The listing builds one solid part. Answer for the finished solid, in the listing's coordinates (mm). A direction names the side the tool comes from. Give positions to 0.01 mm unless a question says otherwise; leave off trailing zeros. Order: outer loops, then holes, each group sorted by start corner. A loop starts at its lowest first (then second) coordinate and runs counter-clockwise, first axis right, second up. Notation, with made-up numbers: (-31.75, -40) - (3.25, -40) arc R34 ccw to (3.25, -4) - close; hole circle Ø11 at (50.5, -8.5). An arc over 180 degrees is marked (long way). Answer as a JSON object with one key per item and string values. Group by question number.
Q1. For faces 1 (the face through (11.923, -3.755, -80.14)), 2 (the face through (11.923, 3.755, 9.86)), 3 (the face through (-0.342, 52.497, -65.07)), determine the directions among +Z, -Z, +X, -X, +Y, -Y from which every point of the face is accessible in a straight line to the end or side of a thin tool.
Q2. A cutting plane is placed at D-D, the plane y = 35. Give the vertices of the cut face in (x, z), and give its area (3 significant figures).
Q3. The mould has two halves that part along Z. Classify faces 4 (the face through (-10, -9, 0)), 5 (the face through (-1.627, 22.606, -34.65)), 6 (the face through (20.188, 21.289, -4.93)), 7 (the face through (1, -9, -10)): released by +Z, released by -Z, zero draft, split by the parting line, or undercut.
Q4. A cutting plane is placed at A-A, the plane y = -2. Give the vertices of the cut face in (x, z).
Q5. A cutting plane is placed at B-B, the plane x = 19.5. Give the vertices of the cut face in (y, z).
Q6. Consider line 1 (Z direction, x = 1, y = 5); line 2 (Z direction, x = 16, y = -31); line 3 (Z direction, x = -2, y = 24). Determine where each line is inside the solid, lowest interval first.
Q7. A cutting plane is placed at C-C, the plane x = 0. Give the vertices of the cut face in (y, z).
Q8. Given pin 1 (8 mm diameter, centred on x = 42, z = -7.5, fed in from +Y); pin 2 (2 mm diameter, centred on x = -12, y = -38, fed in from +Z); pin 3 (12 mm diameter, centred on y = -24.5, z = -74.5, fed in from -X), each flat-ended and moving along its own axis, determine where each tip first touches the part or whether it passes through.
from build123d import *

# Parameters (mm, degrees)
SKETCH2_R           = 12.5
BOSS_EXTRUDE1_DEPTH = 20
BOSS_EXTRUDE2_DEPTH = 10
FILLET1_R           = 5
SKETCH4_R           = 12.5
BOSS_EXTRUDE3_DEPTH = 50
BOSS_EXTRUDE4_START = 20
SKETCH5_R           = 12.5
BOSS_EXTRUDE4_DEPTH = 20


with BuildPart() as part:
    # Sketch2 → Boss-Extrude1 (new body)
    with BuildSketch(Plane.XY):
        Circle(SKETCH2_R)
    extrude(amount=BOSS_EXTRUDE1_DEPTH)

    # Sketch3 → Boss-Extrude2 (add)
    with BuildSketch(Plane.XY):
        with BuildLine():
            Line((-49.999953659, -0.068074118), (-23.953413336, -0.068074118))
            Line((-23.953413336, -0.068074118), (-17.234135678, 38.038843109))
            ThreePointArc((-17.234135678, 38.038843109), (0, 52.5), (17.234135678, 38.038843109))
            Line((17.234135678, 38.038843109), (23.953413336, -0.068074118))
            Line((23.953413336, -0.068074118), (49.999953659, -0.068074118))
            ThreePointArc((49.999953659, -0.068074118), (0, -50), (-49.999953659, -0.068074118))
        make_face()
    boss_extrude2 = extrude(amount=-BOSS_EXTRUDE2_DEPTH)

    # Fillet1
    fillet1_edges = [part.edges().sort_by_distance(p)[0] for p in [
        (-23.953413336, -0.068074118, -5),
        (23.953413336, -0.068074118, -5),
    ]]
    fillet(fillet1_edges, radius=FILLET1_R)

    # Sketch4 → Boss-Extrude3 (add)
    with BuildSketch(Plane(origin=(0, 0, -10), x_dir=(-1, 0, 0), z_dir=(0, 0, -1))):
        with Locations(Location((0, 35, 0), (0, 0, 180))):
            Circle(SKETCH4_R)
    extrude(amount=BOSS_EXTRUDE3_DEPTH)

    # Mirror1: Boss-Extrude2 across plane
    add(boss_extrude2.mirror(Plane(origin=(0, 0, -35), x_dir=(1, 0, 0), z_dir=(0, 0, -1))))

    # Sketch5 → Boss-Extrude4 (add)
    with BuildSketch(Plane(origin=(0, 0, -70), x_dir=(-1, 0, 0), z_dir=(0, 0, -1)).offset(BOSS_EXTRUDE4_START)):
        with Locations(Location((0, 0, 0), (0, 0, 180))):
            Circle(SKETCH5_R)
    extrude(amount=-BOSS_EXTRUDE4_DEPTH)


solid = part.part
Reply:
{
 "1": {"face 1": "-Z", "face 2": "+Z", "face 3": "+Z, -Z, +Y"},
 "2": {"outline": "(-17.77, -70) - (17.77, -70) - (17.77, -60) - (12.5, -60) - (12.5, -10) - (17.77, -10) - (17.77, 0) - (-17.77, 0) - (-17.77, -10) - (-12.5, -10) - (-12.5, -60) - (-17.77, -60) - close", "area": "1,960 mm^2"},
 "3": {"face 4": "released by +Z", "face 5": "undercut", "face 6": "zero draft", "face 7": "undercut"},
 "4": {"outline": "(-49.96, -70) - (-12.34, -70) - (-12.34, -90) - (12.34, -90) - (12.34, -70) - (49.96, -70) - (49.96, -60) - (-49.96, -60) - close; (-49.96, -10) - (49.96, -10) - (49.96, 0) - (12.34, 0) - (12.34, 20) - (-12.34, 20) - (-12.34, 0) - (-49.96, 0) - close"},
 "5": {"outline": "(-46.04, -70) - (25.19, -70) - (25.19, -60) - (-46.04, -60) - close; (-46.04, -10) - (25.19, -10) - (25.19, 0) - (-46.04, 0) - close"},
 "6": {"line 1": "z = -90 to -60, -10 to 20", "line 2": "z = -70 to -60, -10 to 0", "line 3": "z = -70 to 0"},
 "7": {"outline": "(-50, -70) - (-12.5, -70) - (-12.5, -90) - (12.5, -90) - (12.5, -70) - (52.5, -70) - (52.5, -60) - (47.5, -60) - (47.5, -10) - (52.5, -10) - (52.5, 0) - (12.5, 0) - (12.5, 20) - (-12.5, 20) - (-12.5, 0) - (-50, 0) - (-50, -10) - (22.5, -10) - (22.5, -60) - (-50, -60) - close"},
 "8": {"pin 1": "stops at y = -0.07", "pin 2": "stops at z = 0", "pin 3": "stops at x = -45.59"}
}
